Read the model definition and answer for the solid it produces. Units are mm, in the model's axes. Give positions to 0.01 mm unless a question says otherwise; leave off trailing zeros. Loops run counter-clockwise (first coordinate to the right, second up) from the corner with the lowest first, then second, coordinate; pieces in that order, holes last.
(1) Straight lines are drawn through the part: probe 1 along Z at (x, y) = (0.4, 27); probe 2 along Z at (x, y) = (1.05, -48.5); probe 3 along Y at (x, z) = (1.4, 58). For each, find the intervals that lie inside material, in ascending order.
(2) Find section C-C, the plane x = 2.5. State how many separate pieces and enclosed holes the cut face has, then the cut area to 3 significant figures.
(3) Each of these flat-tipped pins is pushed along its axis until it touches: P1, Ø2, axis at x = 2.5, z = 44, coming from the -Y side; P2, Ø1.2, axis at x = 2, y = -4.5, coming from the -Z side; P3, Ø1.5, axis at x = 3.5, y = -18.5, coming from the +Z side. Where does it stop, or does it pass through?
(4) Find section B-B, the plane y = -46. Write down the section's boundary in (x, z), then the cut area to 3 significant figures.
(5) Find section D-D, the plane z = 55. Write down the section's boundary in (x, y).
(6) Find section A-A, the plane z = -70. Write down the section's boundary in (x, y).
```python
from build123d import *

# Parameters (mm, degrees)
SKETCH1_R           = 80
SKETCH1_R_2         = 2
SKETCH1_R_3         = 3
BOSS_EXTRUDE1_DEPTH = 4
SKETCH2_W           = 2.5
SKETCH2_H           = 15
CUT_EXTRUDE1_DEPTH  = 10


with BuildPart() as part:
    # Sketch1 → Boss-Extrude1 (new body)
    with BuildSketch(Plane(origin=(0, 0, 0), x_dir=(0, 0, -1), z_dir=(1, 0, 0))):
        Circle(SKETCH1_R)
        with Locations((0, 17)):
            Circle(SKETCH1_R_2, mode=Mode.SUBTRACT)
        with Locations((0, 35)):
            Circle(SKETCH1_R_2, mode=Mode.SUBTRACT)
        with Locations((0, 70)):
            Circle(SKETCH1_R_2, mode=Mode.SUBTRACT)
        with Locations((70, 0)):
            Circle(SKETCH1_R_2, mode=Mode.SUBTRACT)
        with Locations((35, 0)):
            Circle(SKETCH1_R_2, mode=Mode.SUBTRACT)
        with Locations((0, -70)):
            Circle(SKETCH1_R_2, mode=Mode.SUBTRACT)
        with Locations((0, -35)):
            Circle(SKETCH1_R_2, mode=Mode.SUBTRACT)
        with Locations((-70, 0)):
            Circle(SKETCH1_R_2, mode=Mode.SUBTRACT)
        with Locations((-35, 0)):
            Circle(SKETCH1_R_2, mode=Mode.SUBTRACT)
        with Locations((17, 0)):
            Circle(SKETCH1_R_2, mode=Mode.SUBTRACT)
        with Locations((0, -17)):
            Circle(SKETCH1_R_2, mode=Mode.SUBTRACT)
        Circle(SKETCH1_R_3, mode=Mode.SUBTRACT)
        with Locations((-17, 0)):
            Circle(SKETCH1_R_2, mode=Mode.SUBTRACT)
        with BuildLine():
            Line((-10, 27.886232268), (-10, 58.094750193))
            ThreePointArc((-10, 58.094750193), (-11.938137822, 62.047597268), (-16.25, 62.935979376))
            ThreePointArc((-16.25, 62.935979376), (-45.961940777, 45.961940777), (-62.935979376, 16.25))
            ThreePointArc((-62.935979376, 16.25), (-62.047597268, 11.938137822), (-58.094750193, 10))
            Line((-58.094750193, 10), (-27.886232268, 10))
            ThreePointArc((-27.886232268, 10), (-25.321364567, 10.707977903), (-23.482844729, 12.631418528))
            ThreePointArc((-23.482844729, 12.631418528), (-18.854664285, 18.854664285), (-12.631418528, 23.482844729))
            ThreePointArc((-12.631418528, 23.482844729), (-10.707977903, 25.321364567), (-10, 27.886232268))
        make_face(mode=Mode.SUBTRACT)
        with BuildLine():
            Line((-10, -58.094750193), (-10, -27.886232268))
            ThreePointArc((-10, -27.886232268), (-10.707977903, -25.321364567), (-12.631418528, -23.482844729))
            ThreePointArc((-12.631418528, -23.482844729), (-18.854664285, -18.854664285), (-23.482844729, -12.631418528))
            ThreePointArc((-23.482844729, -12.631418528), (-25.321364567, -10.707977903), (-27.886232268, -10))
            Line((-27.886232268, -10), (-58.094750193, -10))
            ThreePointArc((-58.094750193, -10), (-62.047597268, -11.938137822), (-62.935979376, -16.25))
            ThreePointArc((-62.935979376, -16.25), (-45.961940777, -45.961940777), (-16.25, -62.935979376))
            ThreePointArc((-16.25, -62.935979376), (-11.938137822, -62.047597268), (-10, -58.094750193))
        make_face(mode=Mode.SUBTRACT)
        with BuildLine():
            Line((10, -58.094750193), (10, -27.886232268))
            ThreePointArc((10, -27.886232268), (10.707977903, -25.321364567), (12.631418528, -23.482844729))
            ThreePointArc((12.631418528, -23.482844729), (18.854664285, -18.854664285), (23.482844729, -12.631418528))
            ThreePointArc((23.482844729, -12.631418528), (25.321364567, -10.707977903), (27.886232268, -10))
            Line((27.886232268, -10), (58.094750193, -10))
            ThreePointArc((58.094750193, -10), (62.047597268, -11.938137822), (62.935979376, -16.25))
            ThreePointArc((62.935979376, -16.25), (45.961940777, -45.961940777), (16.25, -62.935979376))
            ThreePointArc((16.25, -62.935979376), (11.938137822, -62.047597268), (10, -58.094750193))
        make_face(mode=Mode.SUBTRACT)
        with BuildLine():
            Line((10, 27.886232268), (10, 58.094750193))
            ThreePointArc((10, 58.094750193), (11.938137822, 62.047597268), (16.25, 62.935979376))
            ThreePointArc((16.25, 62.935979376), (45.961940777, 45.961940777), (62.935979376, 16.25))
            ThreePointArc((62.935979376, 16.25), (62.047597268, 11.938137822), (58.094750193, 10))
            Line((58.094750193, 10), (27.886232268, 10))
            ThreePointArc((27.886232268, 10), (25.321364567, 10.707977903), (23.482844729, 12.631418528))
            ThreePointArc((23.482844729, 12.631418528), (18.854664285, 18.854664285), (12.631418528, 23.482844729))
            ThreePointArc((12.631418528, 23.482844729), (10.707977903, 25.321364567), (10, 27.886232268))
        make_face(mode=Mode.SUBTRACT)
    extrude(amount=BOSS_EXTRUDE1_DEPTH)

    # Sketch2 → Cut-Extrude1 (cut)
    with BuildSketch(Plane.ZY):
        Rectangle(SKETCH2_W, SKETCH2_H)
    extrude(amount=-CUT_EXTRUDE1_DEPTH, mode=Mode.SUBTRACT)


solid = part.part
```
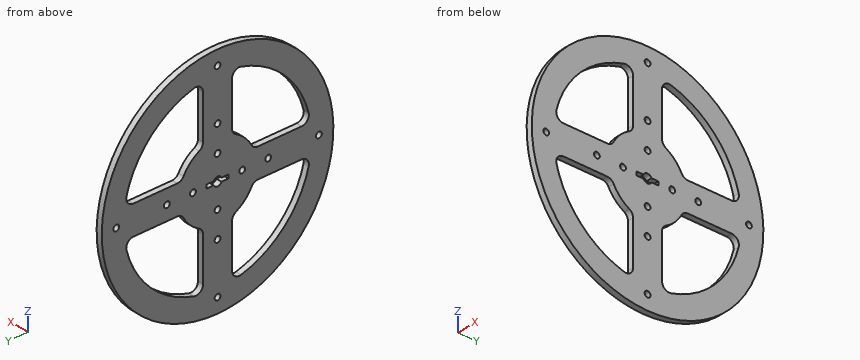
Entries:
1. probe 1: z = -75.31 to -59.13, -10.08 to 10.08, 59.13 to 75.31
1. probe 2: z = -63.62 to -43.28, -10 to 10, 43.28 to 63.62
1. probe 3: y = -55.1 to -29.34, -10 to 10, 29.34 to 55.1
2. separate pieces: 1
2. enclosed holes: 17
2. area: 12,000 mm2
3. P1: stops at y = -67.46
3. P2: stops at z = -79.9
3. P3: stops at z = 78.01
4. outline: (0, -65.45) - (4, -65.45) - (4, -45.92) - (0, -45.92) - close; (0, -10) - (4, -10) - (4, 10) - (0, 10) - close; (0, 45.92) - (4, 45.92) - (4, 65.45) - (0, 65.45) - close
4. area: 236 mm2
5. outline: (0, -58.09) - (4, -58.09) - (4, -34.64) - (0, -34.64) - close; (0, -10) - (4, -10) - (4, 10) - (0, 10) - close; (0, 34.64) - (4, 34.64) - (4, 58.09) - (0, 58.09) - close
6. outline: (0, -38.73) - (4, -38.73) - (4, -2) - (0, -2) - close; (0, 2) - (4, 2) - (4, 38.73) - (0, 38.73) - close
